```python
from build123d import *

# Parameters (mm, degrees)
SKETCH2_W           = 50.8
SKETCH2_H           = 38.1
BOSS_EXTRUDE1_DEPTH = 50.8
SKETCH5_W           = 44.45
SKETCH5_H           = 44.45
CUT_EXTRUDE3_DEPTH  = 82.319677815
SKETCH7_W           = 4.7625
SKETCH7_H           = 25.4
BOSS_EXTRUDE2_DEPTH = 31.75
FILLET1_R           = 5.08
SKETCH8_R           = 4.7625
CUT_EXTRUDE4_DEPTH  = 74.248977169
BOSS_EXTRUDE3_DEPTH = 6.35
SKETCH10_R          = 4.7625
CUT_EXTRUDE5_DEPTH  = 118.96738029
FILLET2_R           = 5.08


with BuildPart() as part:
    # Sketch2 → Boss-Extrude1 (new body)
    with BuildSketch(Plane.XY):
        with Locations((25.4, 19.05)):
            Rectangle(SKETCH2_W, SKETCH2_H)
    extrude(amount=-BOSS_EXTRUDE1_DEPTH)

    # Sketch5 → Cut-Extrude3 (cut, through all)
    with BuildSketch(Plane(origin=(0, 38.1, 0), x_dir=(1, 0, 0), z_dir=(0, 1, 0))):
        with Locations((25.4, 25.4)):
            Rectangle(SKETCH5_W, SKETCH5_H)
    extrude(amount=-CUT_EXTRUDE3_DEPTH, mode=Mode.SUBTRACT)

    # Sketch7 → Boss-Extrude2 (add)
    with BuildSketch(Plane.XY):
        with Locations((15.08125, 12.7)):
            Rectangle(SKETCH7_W, SKETCH7_H)
        with Locations((34.13125, 12.7)):
            Rectangle(SKETCH7_W, SKETCH7_H)
    extrude(amount=BOSS_EXTRUDE2_DEPTH)

    # Fillet1
    fillet1_edges = [part.edges().sort_by_distance(p)[0] for p in [
        (15.08125, 0, 31.75),
        (15.08125, 25.4, 31.75),
        (34.13125, 0, 31.75),
        (34.13125, 25.4, 31.75),
    ]]
    fillet(fillet1_edges, radius=FILLET1_R)

    # Sketch8 → Cut-Extrude4 (cut, through all)
    with BuildSketch(Plane(origin=(36.5125, 0, 0), x_dir=(0, 0, -1), z_dir=(1, 0, 0))):
        with Locations((-19.05, 12.7)):
            Circle(SKETCH8_R)
    extrude(amount=-CUT_EXTRUDE4_DEPTH, mode=Mode.SUBTRACT)

    # Sketch9 → Boss-Extrude3 (add)
    with BuildSketch(Plane(origin=(0, 0, -33.3375), x_dir=(-1, 0, 0), z_dir=(0, 0, -1))):
        Polygon((0, 38.1), (0, 68.2625), (25.4, 68.2625), (25.4, 42.8625), (0, 19.05), align=None)
        Polygon((-76.2, 42.8625), (-50.8, 19.05), (-50.8, 38.1), (-50.8, 68.2625), (-76.2, 68.2625), align=None)
    extrude(amount=-BOSS_EXTRUDE3_DEPTH)

    # Sketch10 → Cut-Extrude5 (cut, through all)
    with BuildSketch(Plane.XY.offset(-26.9875)):
        with Locations((-12.7, 55.5625)):
            Circle(SKETCH10_R)
        with Locations((63.5, 55.5625)):
            Circle(SKETCH10_R)
    extrude(amount=-CUT_EXTRUDE5_DEPTH, mode=Mode.SUBTRACT)

    # Fillet2
    fillet2_edges = [part.edges().sort_by_distance(p)[0] for p in [
        (76.2, 68.2625, -30.1625),
        (50.8, 68.2625, -30.1625),
        (0, 68.2625, -30.1625),
        (-25.4, 68.2625, -30.1625),
    ]]
    fillet(fillet2_edges, radius=FILLET2_R)


solid = part.part
```
Check sheet for the modelled part. Datum: model origin and axes. Units: mm. A direction names the side the tool comes from. Give positions to 0.01 mm unless a question says otherwise; leave off trailing zeros. Order: outer loops, then holes, each group sorted by start corner. A loop starts at its lowest first (then second) coordinate and runs counter-clockwise, first axis right, second up. Notation, with made-up numbers: M -7.75,15.25 L 48.25,15.25 A28 cw 48.25,39.25 Z; hole C 33.5,-9 d10. An arc over 180 degrees is marked long. Answer in a Markdown table with one row per item.
1) Access from +Z, -Z, +X, -X, +Y, -Y to the whole of each face (thin tool, end or side, straight path). Record for faces 4 (the cylindrical face through (-1.449, 66.735, -30.118)), 5 (the flat face through (63.678, 31.123, -30.207)), 6 (the flat face through (3.175, 19, -25)), 7 (the flat face through (25, 19, -50.8)), 8 (the flat face through (34, 25.4, 13)).
Filled sheet:
| item | result |
|---|---|
| face 4 | +Z, -Z, +Y |
| face 5 | +Z, -Z, +X, -Y |
| face 6 | +Y, -Y |
| face 7 | -Z, +X, -X, +Y, -Y |
| face 8 | +Z, +X, -X, +Y |
2) Cross-section at A-A, the plane y = 12.7. Count the separate pieces of the cut face and the enclosed holes in it, plus the area to 3 significant figures.
Filled sheet:
| item | result |
|---|---|
| separate pieces | 3 |
| enclosed holes | 1 |
| area | 817 mm2 |
3) Release check for a two-part mould opening along X. For faces 1 (the cylindrical face through (34.165, 23.951, 30.222)), 2 (the flat face through (17.463, 13, 12)), 3 (the flat face through (36.512, 13, 12)) record: +X half, -X half, draft (parallel to the pull), parting line (faces both ways), or undercut.
Filled sheet:
| item | result |
|---|---|
| face 1 | draft |
| face 2 | undercut |
| face 3 | +X half |
4) Gauge pin test, flat ends, axial feed: P1, Ø4, axis at x = 33.5, z = 17, coming from the +Y side; P2, Ø1, axis at y = 14.5, z = 4, coming from the +X side; P3, Ø7.5, axis at x = 60.5, y = 46.5, coming from the +Z side; P4, Ø19, axis at x = 20, y = 21.5, coming from the +Z side. Record the tip position at first contact, or that the pin passes through.
Filled sheet:
| item | result |
|---|---|
| P1 | stops at y = 25.4 |
| P2 | stops at x = 36.51 |
| P3 | stops at z = -26.99 |
| P4 | stops at z = 31.75 |
5) Cross-section at B-B, the plane x = 24. Enter the section's corners in (y, z) (3 decimals).
Filled sheet:
| item | result |
|---|---|
| outline | M 0,-50.8 L 38.1,-50.8 L 38.1,-47.625 L 0,-47.625 Z; M 0,-3.175 L 38.1,-3.175 L 38.1,0 L 0,0 Z |
6) Thickness scan on L1, parallel to Z at x = 4.5, y = 16.5 (3 decimals); L2, parallel to X at y = 4, z = -4 (3 decimals); L3, parallel to Z at x = 14, y = 12 (3 decimals). Record the ranges inside material, lowest first. Write a range as [from, to].
Filled sheet:
| item | result |
|---|---|
| L1 | z = [-50.8, -47.625], [-3.175, 0] |
| L2 | x = [0, 3.175], [47.625, 50.8] |
| L3 | z = [-50.8, -47.625], [-3.175, 14.339], [23.761, 31.75] |
7) Cross-section at C-C, the plane z = -22.5. Enter the section's corners in (x, y) (3 decimals).
Filled sheet:
| item | result |
|---|---|
| outline | M 0,0 L 3.175,0 L 3.175,38.1 L 0,38.1 Z; M 47.625,0 L 50.8,0 L 50.8,38.1 L 47.625,38.1 Z |
8) Cross-section at D-D, the plane z = 19.05. Enter the section's corners in (x, y).
Filled sheet:
| item | result |
|---|---|
| outline | M 12.7,0 L 17.46,0 L 17.46,7.94 L 12.7,7.94 Z; M 12.7,17.46 L 17.46,17.46 L 17.46,25.4 L 12.7,25.4 Z; M 31.75,0 L 36.51,0 L 36.51,7.94 L 31.75,7.94 Z; M 31.75,17.46 L 36.51,17.46 L 36.51,25.4 L 31.75,25.4 Z |
